Input: dimensioned drawing with shaded views. Units: mm. Origin: part minimum x, y, z. Coordinates: 2 decimals unless noted, no trailing zeros. Order: outer loops, then holes, each group sorted by start corner. A loop starts at its lowest first (then second) coordinate and runs counter-clockwise, first axis right, second up.
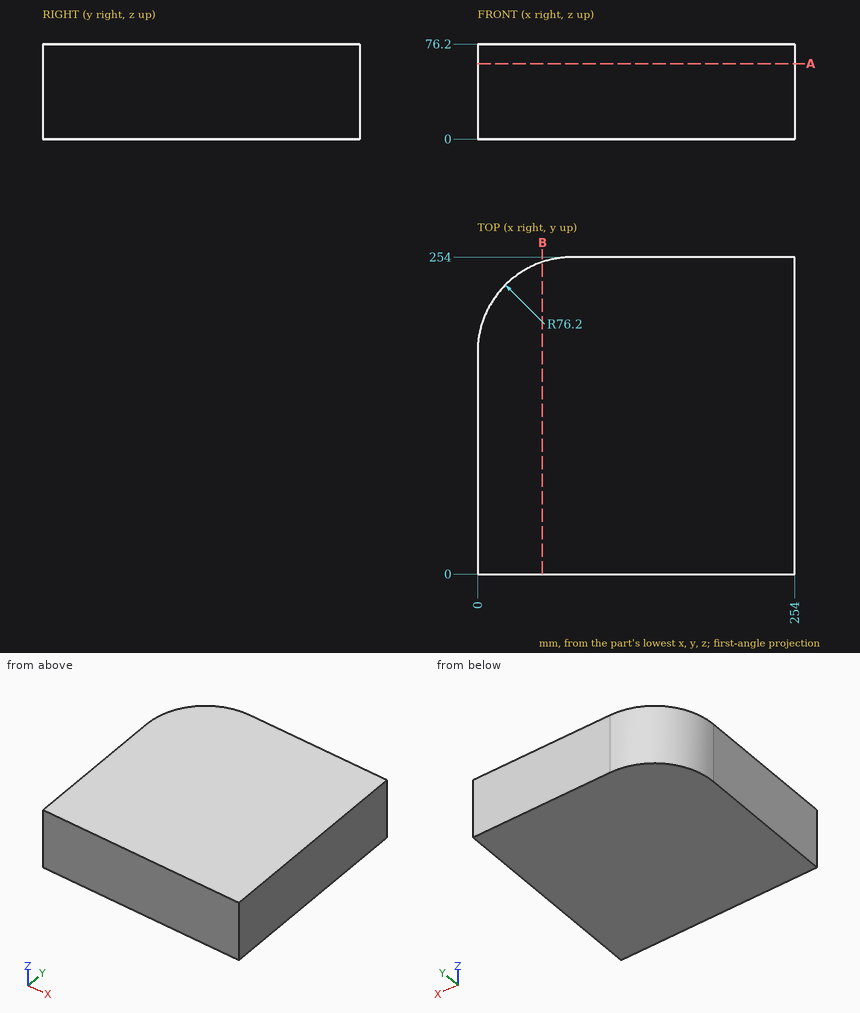
1. Pin query (flat end, axial travel): P1, Ø4, axis at y = 197, z = 60.5, coming from the -X side. Return the tip coordinate at first contact, or that it passes through.
Findings:
P1: stops at x = 1.97
2. Section query B-B on x = 52. Return loops of the section in (y, z).
Findings:
outline: (0, 0) - (250.06, 0) - (250.06, 76.2) - (0, 76.2) - close
3. Ray query, line 1 (X direction, y = 206.5, z = 13); line 2 (Y direction, x = 62, z = 46.5); line 3 (Y direction, x = 58, z = 57.5). Return the intervals inside material, ascending.
Findings:
line 1: x = 5.61 to 254
line 2: y = 0 to 252.67
line 3: y = 0 to 251.79
4. Section query A-A on z = 60.5. Return loops of the section in (x, y), plus the area to 3 significant figures.
Findings:
outline: (0, 0) - (254, 0) - (254, 254) - (76.2, 254) arc R76.2 ccw to (0, 177.8) - close
area: 63,300 mm2
